Geometry: final body of the model. Coordinates: model frame, mm. A direction names the side the tool comes from. Coordinates: 2 decimals unless noted, no trailing zeros. Loops run counter-clockwise (first coordinate to the right, second up) from the corner with the lowest first, then second, coordinate; pieces in that order, holes last. Notation, with made-up numbers: (61, 38.25) -> (81, 38.25) arc R25 cw to (81, 63.25) -> close; hole circle Ø8 at (45.25, -26). An arc over 180 degrees is marked (long way). One line per item, written item: value. Start each with the question number.
Item 1: Mould query, pull axis X, two halves, no side actions, for faces 3 (the cylindrical face through (137.479, 4.378, 126.034)), 4 (the flat face through (139, 9.35, 118)). Classes: +X half, -X half, draft (parallel to the pull), parting line (faces both ways), or undercut.
Item 2: Ray query, probe 1 along Z at (x, y) = (5.5, 4.35); probe 2 along X at (y, z) = (4.25, 130.5); probe 3 along Z at (x, y) = (30, 1.5). Return the intervals inside material, ascending. Write a range as from..to.
Item 3: Section query B-B on y = 13. Return loops of the section in (x, z).
Item 4: Contact query for flat-ended pins moving along their axis: pin 1 Ø4 at (x, z) = (138, 54.5) entering from +Y; pin 2 Ø1.6 at (x, z) = (138, 117) entering from -Y; pin 3 Ø10 at (x, z) = (93.65, 98.77) entering from +Y; pin 4 Ø1.8 at (x, z) = (6.5, 98.5) entering from +Y. Output: stop coordinate, or through.
Item 5: Set-up query: faces 1 (the cylindrical face through (88, 3, 128)), 2 (the cylindrical face through (92.989, 4.822, 118.362)). Return all of +Z, -Z, +X, -X, +Y, -Y with unobstructed straight access to the full face (end or side cutting, diameter ignored); none if empty.
Item 6: Section query A-A on x = 81.1. Return loops of the section in (y, z).
from build123d import *

# Parameters (mm, degrees)
SKETCH1_W                      = 158
SKETCH1_H                      = 199.5
BOSS_EXTRUDE1_DEPTH            = 6.35
BOSS_EXTRUDE2_DEPTH            = 12.7
CBORE_FOR_M4_SHCS1_D           = 4.5
CBORE_FOR_M4_SHCS1_DEPTH       = 6.35
CBORE_FOR_M4_SHCS1_CBORE_D     = 8
CBORE_FOR_M4_SHCS1_CBORE_DEPTH = 4
SKETCH8_R                      = 2.5
ESTOP_DEPTH                    = 7.35
SKETCH9_R                      = 2.5
NUCLEOANDPI_DEPTH              = 7.35
SKETCH10_R                     = 2.7
SKETCH10_R_2                   = 1.2
BUCKS_EXTRUDE_DEPTH            = 3
SKETCH11_R                     = 1.6
BUCKS_CUT_DEPTH                = 6.35
BUCK_2_COUNT                   = 2
BUCK_2_PITCH                   = 28
SKETCH12_R                     = 2.5
PI_2_DEPTH                     = 7.35
SKETCH13_R                     = 1.6
IMU_DEPTH                      = 7.35
SKETCH15_R                     = 3.05
MAGNETS_DEPTH                  = 3.1


with BuildPart() as part:
    # Sketch1 → Boss-Extrude1 (new body)
    with BuildSketch(Plane(origin=(0, 0, 0), x_dir=(1, 0, 0), z_dir=(0, 1, 0))):
        with Locations((79, -99.75)):
            Rectangle(SKETCH1_W, SKETCH1_H)
    extrude(amount=BOSS_EXTRUDE1_DEPTH)

    # Sketch3 → Boss-Extrude2 (add)
    with BuildSketch(Plane(origin=(0, 6.35, 0), x_dir=(1, 0, 0), z_dir=(0, 1, 0))):
        Polygon((158, -199.5), (158, 0), (153, 0), (153, -194.5), (0, -194.5), (0, -199.5), align=None)
    extrude(amount=BOSS_EXTRUDE2_DEPTH)

    # CBORE for M4 SHCS1
    with Locations(Plane(origin=(0, 6.35, 0), x_dir=(1, 0, 0), z_dir=(0, 1, 0))):
        with Locations((138, -55), (20, -179.5), (60, -179.5), (138, -130), (138, -105), (138, -30)):
            CounterBoreHole(CBORE_FOR_M4_SHCS1_D / 2, CBORE_FOR_M4_SHCS1_CBORE_D / 2, CBORE_FOR_M4_SHCS1_CBORE_DEPTH, depth=CBORE_FOR_M4_SHCS1_DEPTH)

    # Sketch8 → eStop (cut, through all)
    with BuildSketch(Plane(origin=(0, 6.35, 0), x_dir=(1, 0, 0), z_dir=(0, 1, 0))):
        with Locations((129.05, -62)):
            Circle(SKETCH8_R)
        with Locations((129.05, -7.75)):
            Circle(SKETCH8_R)
    extrude(amount=-ESTOP_DEPTH, mode=Mode.SUBTRACT)

    # Sketch9 → NucleoAndPi (cut, through all)
    with BuildSketch(Plane(origin=(0, 6.35, 0), x_dir=(1, 0, 0), z_dir=(0, 1, 0))):
        with Locations((16, -15.57)):
            Circle(SKETCH9_R)
        with Locations((81.1, -15.57)):
            Circle(SKETCH9_R)
        with Locations((81.1, -98.77)):
            Circle(SKETCH9_R)
        with Locations((16, -98.77)):
            Circle(SKETCH9_R)
    extrude(amount=-NUCLEOANDPI_DEPTH, mode=Mode.SUBTRACT)

    # Sketch10 → Bucks - Extrude (add)
    with BuildSketch(Plane(origin=(0, 6.35, 0), x_dir=(1, 0, 0), z_dir=(0, 1, 0))):
        with Locations((138, -89)):
            Circle(SKETCH10_R)
        with Locations((138, -89)):
            Circle(SKETCH10_R_2, mode=Mode.SUBTRACT)
        with Locations((107.2, -72)):
            Circle(SKETCH10_R)
        with Locations((107.2, -72)):
            Circle(SKETCH10_R_2, mode=Mode.SUBTRACT)
    bucks_extrude = extrude(amount=BUCKS_EXTRUDE_DEPTH)

    # Sketch11 → Bucks - Cut (cut)
    with BuildSketch(Plane(origin=(0, 6.35, 0), x_dir=(1, 0, 0), z_dir=(0, 1, 0))):
        with Locations((138, -89)):
            Circle(SKETCH11_R)
        with Locations((107.2, -72)):
            Circle(SKETCH11_R)
    bucks_cut = extrude(amount=-BUCKS_CUT_DEPTH, mode=Mode.SUBTRACT)

    # Buck 2: Bucks - Extrude, Bucks - Cut ×2
    with Locations(*[(0, 0, i * BUCK_2_PITCH) for i in range(1, BUCK_2_COUNT)]):
        add(bucks_extrude)
        add(bucks_cut, mode=Mode.SUBTRACT)

    # Sketch12 → Pi 2 (cut, through all)
    with BuildSketch(Plane(origin=(0, 6.35, 0), x_dir=(1, 0, 0), z_dir=(0, 1, 0))):
        with Locations((30, -130.5)):
            Circle(SKETCH12_R)
        with Locations((88, -130.5)):
            Circle(SKETCH12_R)
        with Locations((88, -179.5)):
            Circle(SKETCH12_R)
        with Locations((30, -179.5)):
            Circle(SKETCH12_R)
    extrude(amount=-PI_2_DEPTH, mode=Mode.SUBTRACT)

    # Sketch13 → IMU (cut, through all)
    with BuildSketch(Plane(origin=(0, 6.35, 0), x_dir=(1, 0, 0), z_dir=(0, 1, 0))):
        with Locations((120.22, -159.18)):
            Circle(SKETCH13_R)
        with Locations((120.22, -179.5)):
            Circle(SKETCH13_R)
        with Locations((138, -159.18)):
            Circle(SKETCH13_R)
        with Locations((138, -179.5)):
            Circle(SKETCH13_R)
    extrude(amount=-IMU_DEPTH, mode=Mode.SUBTRACT)

    # Sketch15 → MAGNETS (cut)
    with BuildSketch(Plane(origin=(0, 6.35, 0), x_dir=(1, 0, 0), z_dir=(0, 1, 0))):
        with Locations((5.5, -57.17)):
            Circle(SKETCH15_R)
        with Locations((5.5, -98.77)):
            Circle(SKETCH15_R)
        with Locations((16, -115.385)):
            Circle(SKETCH15_R)
        with Locations((59, -115.385)):
            Circle(SKETCH15_R)
        with Locations((93.65, -98.77)):
            Circle(SKETCH15_R)
        with Locations((93.65, -115.385)):
            Circle(SKETCH15_R)
        with Locations((93.65, -72)):
            Circle(SKETCH15_R)
        with Locations((16, -155)):
            Circle(SKETCH15_R)
    extrude(amount=-MAGNETS_DEPTH, mode=Mode.SUBTRACT)


solid = part.part
Reply:
1. face 3: undercut
1. face 4: draft
2. probe 1: z = 0..54.12, 60.22..95.72, 101.82..199.5
2. probe 2: x = 0..27.5, 32.5..85.5, 90.5..134.03, 141.97..158
2. probe 3: z = 0..128, 133..177, 182..199.5
3. outline: (0, 194.5) -> (153, 194.5) -> (153, 0) -> (158, 0) -> (158, 199.5) -> (0, 199.5) -> close
4. pin 1: stops at y = 2.35
4. pin 2: passes through
4. pin 3: stops at y = 6.35
4. pin 4: stops at y = 3.25
5. face 1: +Y, -Y
5. face 2: +Y
6. outline: (0, 0) -> (6.35, 0) -> (6.35, 13.07) -> (0, 13.07) -> close; (0, 18.07) -> (6.35, 18.07) -> (6.35, 96.27) -> (0, 96.27) -> close; (0, 101.27) -> (6.35, 101.27) -> (6.35, 194.5) -> (19.05, 194.5) -> (19.05, 199.5) -> (0, 199.5) -> close
